from build123d import *

# Parameters (mm, degrees)
F0_W     = 40
F0_H     = 400
F1_DEPTH = 710
F2_W     = 670
F2_H     = 400
F3_DEPTH = 1250
F4_SCALE = 0.1
F5_ANGLE = 180


with BuildPart() as f1:
    # F0 (on Front) → F1 (new body)
    with BuildSketch(Plane.XZ):
        Polygon((0, 50), (0, 0), (40, 0), (1160, 0), (1200, 0), (1200, 50), align=None)
        with Locations((20, -200)):
            Rectangle(F0_W, F0_H)
        with Locations((1180, -200)):
            Rectangle(F0_W, F0_H)
    extrude(amount=F1_DEPTH)

    # F2 (on face) → F3 (cut)
    with BuildSketch(Plane.YZ.offset(1200)):
        with Locations((-355, -200)):
            Rectangle(F2_W, F2_H)
    extrude(amount=-F3_DEPTH, mode=Mode.SUBTRACT)


with BuildPart() as f1_1:
    # F4: moved
    add(f1.part.scale(F4_SCALE))


with BuildPart() as f1_2:
    # F5: moved
    add(f1_1.part.rotate(Axis((0, -35.5, 5), (0, 1, 0)), F5_ANGLE))


solid = f1_2.part
Part model, mm, in its own coordinate system. A direction names the side the tool comes from. Give positions to 0.01 mm unless a question says otherwise; leave off trailing zeros. Loops run counter-clockwise (first coordinate to the right, second up) from the corner with the lowest first, then second, coordinate; pieces in that order, holes last. Notation, with made-up numbers: (-9.5, 49.25) -> (45.5, 49.25) arc R6 cw to (45.5, 56.25) -> close; hole circle Ø8 at (63.25, -24.5). An arc over 180 degrees is marked (long way). Write each question's results on one line, items separated by ' | '. Start each with the question number.
Q1. Band-saw the part on A-A on z = 39.5. List the corners of the cut face in (x, y), plus the area to 3 significant figures.
Q2. Which spindle directions (+Z, -Z, +X, -X, +Y, -Y) get a long thin tool onto all of the face, cutting with end or side? Do faces 1 (the face through (-2, -69, 30)), 2 (the face through (-60, 0, 9)). Say none if no direction does.
Q3. Pull direction Y, two halves, no side cores. Call faces 3 (the face through (-60, -71, 9)), 4 (the face through (-120, -35, 9)), 5 (the face through (-2, -2, 30)): +Y half, -Y half, draft (parallel to the pull), parting line (faces both ways), or undercut.
Q4. Wall check: L1, parallel to Z at x = -44, y = -11.5. Give the ranges that are in metal, low to high.
Q5. Band-saw the part on C-C on y = -15.5. List the corners of the cut face in (x, z).
Q6. Band-saw the part on B-B on x = -7. List the corners of the cut face in (y, z), plus the area to 3 significant figures.
Results are:
1) outline: (-120, -71) -> (-116, -71) -> (-116, -69) -> (-120, -69) -> close; (-120, -2) -> (-116, -2) -> (-116, 0) -> (-120, 0) -> close; (-4, -71) -> (0, -71) -> (0, -69) -> (-4, -69) -> close; (-4, -2) -> (0, -2) -> (0, 0) -> (-4, 0) -> close | area: 32.0 mm²
2) face 1: +Z, +X, -X | face 2: +Z, -Z, +X, -X, +Y
3) face 3: -Y half | face 4: draft | face 5: undercut
4) L1: z = 5 to 10
5) outline: (-120, 5) -> (0, 5) -> (0, 10) -> (-120, 10) -> close
6) outline: (-71, 5) -> (0, 5) -> (0, 10) -> (-71, 10) -> close | area: 355 mm²
